from build123d import *

# Parameters (mm, degrees)
F0_W          = 64.262
F0_H          = 35.306
F0_W_2        = 61.722
F0_H_2        = 32.766
F1_DEPTH      = 25.4
F2_W          = 66.802
F2_H          = 37.846
F2_W_2        = 64.262
F2_H_2        = 35.306
F3_DEPTH      = 1.778
F3_DEPTH_BACK = 25.4


with BuildPart() as f1:
    # F0 (on Top) → F1 (new body)
    with BuildSketch(Plane.XY):
        Rectangle(F0_W, F0_H)
        Rectangle(F0_W_2, F0_H_2, mode=Mode.SUBTRACT)
    extrude(amount=-F1_DEPTH)

    # F2 (on Top) → F3 (join, two sides)
    with BuildSketch(Plane.XY) as f3_sk:
        Rectangle(F2_W, F2_H)
        Rectangle(F2_W_2, F2_H_2, mode=Mode.SUBTRACT)
    extrude(amount=F3_DEPTH)
    extrude(f3_sk.sketch, amount=-F3_DEPTH_BACK)


solid = f1.part
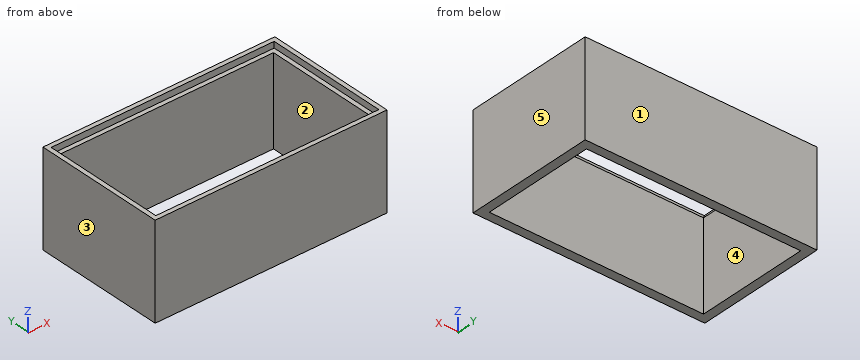
Can you work these out from the model? Positions are in its coordinate system, mm. Face numbers are marked on the shaded views. A direction names the side the tool comes from. Round coordinates to 2 decimals unless told otherwise and drop trailing zeros. Order: outer loops, then holes, each group sorted by start corner. A loop starts at its lowest first (then second) coordinate and runs counter-clockwise, first axis right, second up. Notation, with made-up numbers: (-10, 46.25) - (12, 46.25) arc R25 cw to (12, 84.25) - close; hole circle Ø8 at (11, -23). An arc over 180 degrees is marked (long way). Answer in a Markdown table with one row per item.
(1) Suppose I cut it at A-A, the plane y = -3. Please give me the cut outline in (x, z).
From the geometry:
| item | result |
|---|---|
| outline | (-33.4, -25.4) - (-30.86, -25.4) - (-30.86, 0) - (-32.13, 0) - (-32.13, 1.78) - (-33.4, 1.78) - close; (30.86, -25.4) - (33.4, -25.4) - (33.4, 1.78) - (32.13, 1.78) - (32.13, 0) - (30.86, 0) - close |
(2) Suppose I cut it at C-C, the plane z = -22. Please give me the cut outline in (x, y), plus the area to 3 significant figures.
From the geometry:
| item | result |
|---|---|
| outline | (-33.4, -18.92) - (33.4, -18.92) - (33.4, 18.92) - (-33.4, 18.92) - close; hole (-30.86, -16.38) - (30.86, -16.38) - (30.86, 16.38) - (-30.86, 16.38) - close |
| area | 506 mm2 |
(3) Which directions (+Z, -Z, +X, -X, +Y, -Y) give clear straight access to the entire face, cutting with the end or side of a thin tool? Please do the marked faces 1 and 2.
From the geometry:
| item | result |
|---|---|
| face 1 | +Z, -Z, +X, -X, +Y |
| face 2 | +Z, -Z |
(4) Please list where these lines run through material, in increasing order: L1, parallel to Y at x = 21, z = -13; L2, parallel to X at y = -4, z = -3.5; L3, parallel to Z at x = 16, y = 17. Write a range as from..to.
From the geometry:
| item | result |
|---|---|
| L1 | y = -18.92..-16.38, 16.38..18.92 |
| L2 | x = -33.4..-30.86, 30.86..33.4 |
| L3 | z = -25.4..0 |
(5) If we mould it in two halves opening along X, with no side actions, what happens to the marked faces 3, 4 and 5? For each: released by +X, released by -X, zero draft, split by the parting line, or undercut.
From the geometry:
| item | result |
|---|---|
| face 3 | released by -X |
| face 4 | undercut |
| face 5 | released by +X |
(6) Suppose I cut it at B-B, the plane x = -3. Please give me the cut outline in (y, z), plus the area to 3 significant figures.
From the geometry:
| item | result |
|---|---|
| outline | (-18.92, -25.4) - (-16.38, -25.4) - (-16.38, 0) - (-17.65, 0) - (-17.65, 1.78) - (-18.92, 1.78) - close; (16.38, -25.4) - (18.92, -25.4) - (18.92, 1.78) - (17.65, 1.78) - (17.65, 0) - (16.38, 0) - close |
| area | 134 mm2 |
